from build123d import *

# Parameters (mm, degrees)
BOSS_EXTRUDE1_DEPTH = 4.8
SKETCH3_W           = 0.3
SKETCH3_H           = 1.6
CUT_EXTRUDE1_DEPTH  = 114.8
CUT_EXTRUDE2_DEPTH  = 114.8


with BuildPart() as part:
    # Sketch2 → Boss-Extrude1 (new body)
    with BuildSketch(Plane(origin=(0, 0, 0), x_dir=(1, 0, 0), z_dir=(0, 1, 0))):
        with BuildLine():
            Line((-16.5, -21), (16.5, -21))
            ThreePointArc((16.5, -21), (18.621320344, -20.121320344), (19.5, -18))
            Line((19.5, -18), (19.5, 18))
            ThreePointArc((19.5, 18), (18.621320344, 20.121320344), (16.5, 21))
            Line((16.5, 21), (-16.5, 21))
            ThreePointArc((-16.5, 21), (-18.621320344, 20.121320344), (-19.5, 18))
            Line((-19.5, 18), (-19.5, -18))
            ThreePointArc((-19.5, -18), (-18.621320344, -20.121320344), (-16.5, -21))
        make_face()
    extrude(amount=BOSS_EXTRUDE1_DEPTH)

    # Sketch3 → Cut-Extrude1 (cut)
    with BuildSketch(Plane.XY.offset(21)):
        Polygon((-16.5, 1.3), (-16.5, 2.9), (-17.9, 2.9), (-19.5, 2.9), (-19.5, 1.3), (-19.5, 0), (-17.9, 0), (-17.9, 1.3), align=None)
        Polygon((17.9, 2.9), (16.5, 2.9), (16.5, 1.3), (17.9, 1.3), (17.9, 0), (19.5, 0), (19.5, 1.3), (19.5, 2.9), align=None)
        with Locations((-16.35, 2.1)):
            Rectangle(SKETCH3_W, SKETCH3_H)
        with Locations((16.35, 2.1)):
            Rectangle(SKETCH3_W, SKETCH3_H)
    extrude(amount=-CUT_EXTRUDE1_DEPTH, mode=Mode.SUBTRACT)

    # Sketch4 → Cut-Extrude2 (cut)
    with BuildSketch(Plane.ZY.offset(19.5)):
        Polygon((17.5, 2.9), (21, 2.9), (21, 1.2), (21, 0), (19.25, 0), (19.25, 1.3), (17.5, 1.3), align=None)
    extrude(amount=-CUT_EXTRUDE2_DEPTH, mode=Mode.SUBTRACT)


solid = part.part
Build history of the part. All positions in model axes, mm. A direction names the side the tool comes from. Coordinates: 2 decimals unless noted, no trailing zeros. Write each loop counter-clockwise with the first axis right and the second up, starting at its lowest first coordinate (ties: lowest second). Pieces come first, ordered by that corner, then holes. Notation, with made-up numbers: (47.25, 24) -> (58.25, 24) arc R25 cw to (58.25, 59) -> close; hole circle Ø4 at (-0.75, 88). An arc over 180 degrees is marked (long way). Use CSV: the item, a comma, the result in double quotes. Start each with the question number.
Q1. Flat gauge pins, fed straight in: pin 1 Ø0.5 at (y, z) = (2, 5.5) entering from +X; pin 2 Ø1.4 at (y, z) = (1, -10.5) entering from -X; pin 3 Ø0.8 at (x, y) = (6, 2) entering from +Z. Where does each tip first touch, or does it go through?
Q2. Cut at C-C, the plane x = -17. List the corners of the cut face in (y, z), then the cut area to 3 significant figures.
Q3. Pull direction Y, two halves, no side cores. Call faces 1 (the flat face through (0, 0, -1)), 2 (the cylindrical face through (-17.211, 0.641, -20.914)), 3 (the flat face through (0, 1.3, 19)), 4 (the flat face through (-16.2, 2, -1)): released by +Y, released by -Y, zero draft, split by the parting line, or undercut.
Q4. Cut at A-A, the plane x = 5. List the corners of the cut face in (y, z).
Q5. 3-axis set-ups, long thin cutter, end or side, ignore diameter. For faces 5 (the flat face through (-17.9, 1, 0)), 6 (the flat face through (0, 1, 19.25)), 7 (the flat face through (1, 2.9, 19)), 8 (the flat face through (0, 2, 17.5)): which of +Z, -Z, +X, -X, +Y, -Y reach the whole face in a straight line?
Q6. Drill centre lines: probe 1 along Y at (x, z) = (17.5, 1); probe 2 along X at (y, z) = (2.8, -12); probe 3 along Y at (x, z) = (12, 19.5). Where is each one in solid material? Low to high.
Q7. Cut at B-B, the plane z = -4.5. List the corners of the cut face in (x, y), then the cut area to 3 significant figures.
Q8. Cut at D-D, the plane y = 0.65. List the corners of the cut face in (x, z), then the cut area to 3 significant figures.
Checked values:
1,pin 1,"stops at x = 16.2"
1,pin 2,"stops at x = -17.9"
1,pin 3,"stops at z = 17.5"
2,outline,"(0, -20.96) -> (1.3, -20.96) -> (1.3, 19.25) -> (0, 19.25) -> close; (2.9, -20.96) -> (4.8, -20.96) -> (4.8, 20.96) -> (2.9, 20.96) -> close"
2,area,"132 mm²"
3,face 1,"released by -Y"
3,face 2,"zero draft"
3,face 3,"undercut"
3,face 4,"undercut"
4,outline,"(0, -21) -> (4.8, -21) -> (4.8, 21) -> (2.9, 21) -> (2.9, 17.5) -> (1.3, 17.5) -> (1.3, 19.25) -> (0, 19.25) -> close"
5,face 5,"+Z, -Z, -X, -Y"
5,face 6,"+Z, +X, -X, -Y"
5,face 7,"+Z"
5,face 8,"+Z, +X, -X"
6,probe 1,"y = 0 to 1.3, 2.9 to 4.8"
6,probe 2,"x = -16.2 to 16.2"
6,probe 3,"y = 2.9 to 4.8"
7,outline,"(-19.5, 2.9) -> (-16.2, 2.9) -> (-16.2, 1.3) -> (-17.9, 1.3) -> (-17.9, 0) -> (17.9, 0) -> (17.9, 1.3) -> (16.2, 1.3) -> (16.2, 2.9) -> (19.5, 2.9) -> (19.5, 4.8) -> (-19.5, 4.8) -> close"
7,area,"172 mm²"
8,outline,"(-17.9, -20.65) arc R3 ccw to (-16.5, -21) -> (16.5, -21) arc R3 ccw to (17.9, -20.65) -> (17.9, 19.25) -> (-17.9, 19.25) -> close"
8,area,"1,440 mm²"
